Design review of the part built by this model. Coordinates are the model's own, in mm. A direction names the side the tool comes from. Give positions to 0.01 mm unless a question says otherwise; leave off trailing zeros. Write each loop counter-clockwise with the first axis right and the second up, starting at its lowest first coordinate (ties: lowest second). Pieces come first, ordered by that corner, then holes. Notation, with made-up numbers: (-3.75, 59.25) -> (18.25, 59.25) arc R26 ccw to (18.25, 92.25) -> close; hole circle Ø11 at (-23.5, 67). An arc over 180 degrees is marked (long way). Answer as a JSON object with one key per item and string values.
```python
from build123d import *

# Parameters (mm, degrees)
F0_R     = 7
F1_DEPTH = 21.5


with BuildPart() as f1:
    # F0 (on Front) → F1 (new body, symmetric)
    with BuildSketch(Plane.XZ):
        with BuildLine():
            Line((-14, 11), (-14, -7))
            Line((-14, -7), (-7, -14))
            Line((-7, -14), (20.601225, -14))
            ThreePointArc((20.601225, -14), (23.892034, -15.235617), (25.556371, -18.331769))
            ThreePointArc((25.556371, -18.331769), (27.745149, -26.119689), (32, -33))
            Line((32, -33), (38, -33))
            Line((38, -33), (67, 0))
            Line((67, 0), (67, 19))
            Line((67, 19), (62, 24))
            Line((62, 24), (38, 24))
            ThreePointArc((38, 24), (29.574973, 16.276069), (18.243085, 14.783252))
            Line((18.243085, 14.783252), (0, 18))
            Line((0, 18), (-7, 18))
            Line((-7, 18), (-14, 11))
        make_face()
        Circle(F0_R, mode=Mode.SUBTRACT)
    extrude(amount=F1_DEPTH, both=True)


solid = f1.part
```
(1) For line 1 along Z through (x, y) = (0, -13); line 2 along Z through (x, y) = (4.5, 6.5); line 3 along X through (y, z) = (7.5, -6), list the stretches that pass through material, from the lowest coordinate up.
Here are the results:
{"line 1": "z = -14 to -7, 7 to 18", "line 2": "z = -14 to -5.36, 5.36 to 17.21", "line 3": "x = -14 to -3.61, 3.61 to 61.73"}
(2) We need section D-D, the plane z = -15. State the section outline as (x, y) points, then the cut area to 3 significant figures.
Here are the results:
{"outline": "(23.6, -21.5) -> (53.82, -21.5) -> (53.82, 21.5) -> (23.6, 21.5) -> close", "area": "1,300 mm²"}
(3) For faces 5 (the flat face through (9.25, -0.3, 16.37)), 6 (the flat face through (-3, 0, 18)), 7 (the flat face through (-14, 0, 2)), list the 3-axis set-ups (+Z, -Z, +X, -X, +Y, -Y) from which the entire face can be reached by the end or side of a thin tool; tool diameter is ignored.
Here are the results:
{"face 5": "+Z, +Y, -Y", "face 6": "+Z, -X, +Y, -Y", "face 7": "+Z, -Z, -X, +Y, -Y"}
(4) We need section C-C, the plane x = 12. State the section outline as (y, z) points, then the cut area to 3 significant figures.
Here are the results:
{"outline": "(-21.5, -14) -> (21.5, -14) -> (21.5, 15.88) -> (-21.5, 15.88) -> close", "area": "1,290 mm²"}
(5) The part is to be moulded in two halves that separate along X. For faces 1 (the cylindrical face through (6.466, 0.301, -2.681)), 2 (the cylindrical face through (23.85, -0.3, -15.2)), 3 (the flat face through (52.3, -0.3, -16.73)), 4 (the flat face through (7, 0, -14)), say which applies: +X half, -X half, draft (parallel to the pull), parting line (faces both ways), or undercut.
Here are the results:
{"face 1": "undercut", "face 2": "-X half", "face 3": "+X half", "face 4": "draft"}
(6) We need section A-A, the plane y = -5.5. State the section outline as (x, z) points, then the cut area to 3 significant figures.
Here are the results:
{"outline": "(-14, -7) -> (-7, -14) -> (20.6, -14) arc R5 cw to (25.56, -18.33) arc R29 ccw to (32, -33) -> (38, -33) -> (67, 0) -> (67, 19) -> (62, 24) -> (38, 24) arc R19 cw to (18.24, 14.78) -> (0, 18) -> (-7, 18) -> (-14, 11) -> close; hole circle Ø14 at (0, 0)", "area": "2,780 mm²"}
(7) We need section B-B, the plane z = 2. State the section outline as (x, y) points, then the cut area to 3 significant figures.
Here are the results:
{"outline": "(-14, -21.5) -> (-6.71, -21.5) -> (-6.71, 21.5) -> (-14, 21.5) -> close; (6.71, -21.5) -> (67, -21.5) -> (67, 21.5) -> (6.71, 21.5) -> close", "area": "2,910 mm²"}
(8) Clearance check with flat-ended pins moving along their axes: pin 1 (2 mm diameter, centred on y = -12.5, z = -25.5, fed in from -X); pin 2 (6 mm diameter, centred on y = -15.5, z = -24, fed in from -X); pin 3 (14 mm diameter, centred on x = 11, y = -2, fed in from -Z). State where each tip first meets the part, or that it passes through.
Here are the results:
{"pin 1": "stops at x = 27.09", "pin 2": "stops at x = 26.04", "pin 3": "stops at z = -14"}
